```python
from build123d import *

# Parameters (mm, degrees)
SKETCH1_R  = 0.85
BODY_DEPTH = 1
FILLET1_R  = 0.2
FILLET2_R  = 0.5


with BuildPart() as part:
    # Sketch1 → Body (new body)
    with BuildSketch(Plane.XY):
        with BuildLine():
            Line((-1, -8.406045209), (-1, -12.227002197))
            ThreePointArc((-1, -12.227002197), (-2.901836737, -11.902811864), (-4.724092893, -11.269199328))
            Line((-4.724092893, -11.269199328), (-5.275907107, -8.139705412))
            ThreePointArc((-5.275907107, -8.139705412), (0, 9.7), (5.275907107, -8.139705412))
            Line((5.275907107, -8.139705412), (4.724092893, -11.269199328))
            ThreePointArc((4.724092893, -11.269199328), (2.901836737, -11.902811864), (1, -12.227002197))
            Line((1, -12.227002197), (1, -8.406045209))
            ThreePointArc((1, -8.406045209), (0, 7.23), (-1, -8.406045209))
        make_face()
        with Locations((3, -9.844424101)):
            Circle(SKETCH1_R, mode=Mode.SUBTRACT)
        with Locations((-3, -9.844424101)):
            Circle(SKETCH1_R, mode=Mode.SUBTRACT)
    extrude(amount=-BODY_DEPTH)

    # Fillet1
    fillet1_edges = [part.edges().sort_by_distance(p)[0] for p in [
        (-4.724092893, -11.269199328, -0.5),
        (4.724092893, -11.269199328, -0.5),
    ]]
    fillet(fillet1_edges, radius=FILLET1_R)

    # Fillet2
    fillet2_edges = [part.edges().sort_by_distance(p)[0] for p in [
        (-5.275907107, -8.139705412, -0.5),
        (5.275907107, -8.139705412, -0.5),
    ]]
    fillet(fillet2_edges, radius=FILLET2_R)


solid = part.part
```
Check sheet for the modelled part. Datum: model origin and axes. Units: mm. A direction names the side the tool comes from. Round coordinates to 2 decimals unless told otherwise and drop trailing zeros. Order: outer loops, then holes, each group sorted by start corner. A loop starts at its lowest first (then second) coordinate and runs counter-clockwise, first axis right, second up. Notation, with made-up numbers: M 73.25,74 L 87.25,74 A20 cw 87.25,90 Z; hole C 4.25,1.5 d5. An arc over 180 degrees is marked long. Answer in a Markdown table with one row per item.
(1) Section check D-D on x = -6.5. Record the boundary of the cut face in (y, z), plus the area to 3 significant figures.
Findings:
| item | result |
|---|---|
| outline | M -7.2,-1 L -5.02,-1 L -5.02,0 L -7.2,0 Z; M 3.78,-1 L 7.2,-1 L 7.2,0 L 3.78,0 Z |
| area | 5.60 mm^2 |
(2) Gauge pin test, flat end, axial feed: pin 1 (0.5 mm diameter, centred on y = -10.5, z = -0.5, fed in from +X). Record the tip position at first contact, or that the pin passes through.
Findings:
| item | result |
|---|---|
| pin 1 | stops at x = 4.9 |
(3) Section check A-A on y = -0.62. Record the boundary of the cut face in (x, z).
Findings:
| item | result |
|---|---|
| outline | M -9.68,-1 L -7.85,-1 L -7.85,0 L -9.68,0 Z; M 7.85,-1 L 9.68,-1 L 9.68,0 L 7.85,0 Z |
(4) Section check C-C on z = -0.8. Record the boundary of the cut face in (x, y).
Findings:
| item | result |
|---|---|
| outline | M -5.45,-8.02 A0.5 cw -5.24,-8.35 L -4.74,-11.16 A0.2 ccw -4.63,-11.31 A11.65 ccw -1,-12.23 L -1,-8.41 A7.85 cw long 1,-8.41 L 1,-12.23 A11.65 ccw 4.63,-11.31 A0.2 ccw 4.74,-11.16 L 5.24,-8.35 A0.5 cw 5.45,-8.02 A9.7 ccw long Z; hole C -3,-9.84 d1.7; hole C 3,-9.84 d1.7 |
(5) Set-up check for faces 1 (the cylindrical face through (-2.824, -11.923, -0.493)), 2 (the flat face through (-1, -10.3, -0.5)): record each of +Z, -Z, +X, -X, +Y, -Y from which the full face is reachable in a straight line by a thin tool's end or side.
Findings:
| item | result |
|---|---|
| face 1 | +Z, -Z, -X, -Y |
| face 2 | +Z, -Z, -Y |
(6) Section check B-B on x = 3. Record the boundary of the cut face in (y, z).
Findings:
| item | result |
|---|---|
| outline | M -11.88,-1 L -10.69,-1 L -10.69,0 L -11.88,0 Z; M -8.99,-1 L -7.87,-1 L -7.87,0 L -8.99,0 Z; M 6.63,-1 L 9.22,-1 L 9.22,0 L 6.63,0 Z |
(7) Material ranges on line 1 along Y through (x, z) = (3, -0.3); line 2 along X through (y, z) = (-10.5, -0.45); line 3 along X through (y, z) = (-1.25, -0.8), recorded low to high. Write a range as from..to.
Findings:
| item | result |
|---|---|
| line 1 | y = -11.88..-10.69, -8.99..-7.87, 6.63..9.22 |
| line 2 | x = -4.86..-3.54, -2.46..-1, 1..2.46, 3.54..4.86 |
| line 3 | x = -9.62..-7.82, 7.82..9.62 |
(8) Draft check along X on faces 3 (the flat face through (5, -9.7, -0.5)), 4 (the cylindrical face through (2.816, -10.674, -0.493)), 5 (the cylindrical face through (-0.346, 9.694, -0.493)), 6 (the flat face through (1, -10.3, -0.5)). Enter one of: +X half, -X half, draft (parallel to the pull), parting line (faces both ways), or undercut.
Findings:
| item | result |
|---|---|
| face 3 | +X half |
| face 4 | undercut |
| face 5 | parting line |
| face 6 | undercut |
